Source: CAD feature listing. Evaluate the final solid. Frame: model axes, mm. A direction names the side the tool comes from. Coordinates: 2 decimals unless noted, no trailing zeros. Write each loop counter-clockwise with the first axis right and the second up, starting at its lowest first coordinate (ties: lowest second). Pieces come first, ordered by that corner, then holes. Notation, with made-up numbers: M 44,9.5 L 98,9.5 A15 cw 98,22.5 Z; hole C 22.25,-19 d1. An arc over 180 degrees is marked long. Answer as CSV lines item,"result". Start each with the question number.
1. Section C-C on y = -10. Return the cut outline in (x, z), plus the area to 3 significant figures.
2. Line query: probe 1 along Y at (x, z) = (-26, -24); probe 2 along X at (y, z) = (-25, -14.5); probe 3 along X at (y, z) = (11, -19.5). Output: solid intervals per line, ascending. Write a range as [from, to].
3. Contact query for flat-ended pins moving along their axis: pin 1 Ø1.5 at (x, z) = (12, 3) entering from -Y; pin 2 Ø7 at (x, y) = (-24.5, -17.5) entering from +Z; pin 3 Ø3 at (y, z) = (11.5, -17.5) entering from +X. Output: stop coordinate, or through.
4. Section D-D on z = -43.5. Return the cut outline in (x, y), plus the area to 3 significant figures.
5. Section A-A on z = -24. Return the cut outline in (x, y), plus the area to 3 significant figures.
6. Reachability of faces 5 (the face through (0, 4, -50)), 6 (the face through (-20.5, -26.3, -24.1)), 7 (the face through (50, 3, 6.5)), 8 (the face through (-37.5, 10, -24)) from +Z, -Z, +X, -X, +Y, -Y: full face, straight path, thin tool, end or side. Return the list, or none.
7. Mould query, pull axis Y, two halves, no side actions, for faces 1 (the face through (-31, -26, -28)), 2 (the face through (10, 0, -2)), 3 (the face through (-40.5, 7, -21)), 4 (the face through (1, 5, -13)). Classes: pulls with the +Y half, pulls with the -Y half, needs draft (parallel to the pull), parting line crosses it, or undercut.
8. Section B-B on x = 54. Return the cut outline in (y, z).
```python
from build123d import *

# Parameters (mm, degrees)
EXTRUDE_1_DEPTH     = 5
SKETCH_2_W          = 20
SKETCH_2_H          = 72
EXTRUDE_2_DEPTH     = 33
SKETCH_3_R          = 3
CUT_EXTRUDE_1_DEPTH = 30
SKETCH_4_R          = 5
CUT_EXTRUDE_2_DEPTH = 17
EXTRUDE_START       = 3
SKETCH_5_R          = 5
EXTRUDE_3_DEPTH     = 3
EXTRUDE_4_DEPTH     = 3
EXTRUDE_5_DEPTH     = 10
SKETCH_8_W          = 42
SKETCH_8_H          = 5
EXTRUDE_6_DEPTH     = 25
CUT_EXTRUDE_3_DEPTH = 10
SKETCH_10_W         = 75
SKETCH_10_H         = 0.5
CUT_EXTRUDE_4_DEPTH = 0.5
SKETCH_11_W         = 0.5
SKETCH_11_H         = 15
SKETCH_11_H_2       = 48
CUT_EXTRUDE_5_DEPTH = 0.5


with BuildPart() as part:
    # 草图1 → 凸台-拉伸1 (new body)
    with BuildSketch(Plane(origin=(0, 0, 0), x_dir=(1, 0, 0), z_dir=(0, 1, 0))):
        Polygon((-37.5, 76), (-37.5, -26), (37.5, -26), (37.5, 16), (0, 16), (0, 76), align=None)
    extrude(amount=EXTRUDE_1_DEPTH)

    # 草图2 → 凸台-拉伸2 (add)
    with BuildSketch(Plane.XZ):
        with Locations((-27.5, -40)):
            Rectangle(SKETCH_2_W, SKETCH_2_H)
    extrude(amount=EXTRUDE_2_DEPTH)

    # 草图3 → 切除-拉伸1 (cut)
    with BuildSketch(Plane.ZY.offset(37.5)):
        with Locations((-56, -23)):
            Circle(SKETCH_3_R)
        with Locations((-24, -23)):
            Circle(SKETCH_3_R)
    extrude(amount=-CUT_EXTRUDE_1_DEPTH, mode=Mode.SUBTRACT)

    # 草图4 → 切除-拉伸2 (cut)
    with BuildSketch(Plane.ZY.offset(37.5)):
        with Locations((-56, -23)):
            Circle(SKETCH_4_R)
        with Locations((-24, -23)):
            Circle(SKETCH_4_R)
    extrude(amount=-CUT_EXTRUDE_2_DEPTH, mode=Mode.SUBTRACT)

    # 草图5 → 凸台-拉伸3 (add)
    with BuildSketch(Plane.ZY.offset(37.5).offset(EXTRUDE_START)):
        Polygon((-76, 5), (26, 5), (26, 0), (-4, 0), (-4, -33), (-76, -33), align=None)
        with Locations((-56, -23)):
            Circle(SKETCH_5_R, mode=Mode.SUBTRACT)
        with Locations((-24, -23)):
            Circle(SKETCH_5_R, mode=Mode.SUBTRACT)
    extrude(amount=-EXTRUDE_3_DEPTH)

    # 草图6 → 凸台-拉伸4 (add)
    with BuildSketch(Plane(origin=(0, 0, -76), x_dir=(-1, 0, 0), z_dir=(0, 0, -1))):
        Polygon((0, 5), (0, 0), (17.5, 0), (17.5, -33), (40.5, -33), (40.5, 5), align=None)
    extrude(amount=EXTRUDE_4_DEPTH)

    # 草图7 → 凸台-拉伸5 (add)
    with BuildSketch(Plane(origin=(0, 5, 0), x_dir=(1, 0, 0), z_dir=(0, 1, 0))):
        Polygon((0, 76), (0, 79), (-40.5, 79), (-40.5, -26), (-37.5, -26), (-37.5, 76), align=None)
    extrude(amount=EXTRUDE_5_DEPTH)

    # 草图8 → 凸台-拉伸6 (add)
    with BuildSketch(Plane(origin=(37.5, 0, 0), x_dir=(0, 0, -1), z_dir=(1, 0, 0))):
        with Locations((-5, 2.5)):
            Rectangle(SKETCH_8_W, SKETCH_8_H)
    extrude(amount=EXTRUDE_6_DEPTH)

    # 草图9 → 切除-拉伸3 (cut)
    with BuildSketch(Plane(origin=(0, 5, 0), x_dir=(1, 0, 0), z_dir=(0, 1, 0))):
        with BuildLine():
            Line((57.5, -3.5), (42.5, -3.5))
            ThreePointArc((42.5, -3.5), (41, -5), (42.5, -6.5))
            Line((42.5, -6.5), (57.5, -6.5))
            ThreePointArc((57.5, -6.5), (59, -5), (57.5, -3.5))
        make_face()
    extrude(amount=-CUT_EXTRUDE_3_DEPTH, mode=Mode.SUBTRACT)

    # 草图10 → 切除-拉伸4 (cut)
    with BuildSketch(Plane.ZY.offset(40.5)):
        with Locations((-41.5, -0.25)):
            Rectangle(SKETCH_10_W, SKETCH_10_H)
    extrude(amount=-CUT_EXTRUDE_4_DEPTH, mode=Mode.SUBTRACT)

    # 草图11 → 切除-拉伸5 (cut)
    with BuildSketch(Plane.ZY.offset(40.5)):
        with Locations((-3.75, 7.5)):
            Rectangle(SKETCH_11_W, SKETCH_11_H)
        with Locations((-38.75, -9)):
            Rectangle(SKETCH_11_W, SKETCH_11_H_2)
    extrude(amount=-CUT_EXTRUDE_5_DEPTH, mode=Mode.SUBTRACT)


solid = part.part
```
Values:
1,outline,"M -40.5,-79 L -17.5,-79 L -17.5,-4 L -40.5,-4 L -40.5,-38.5 L -40,-38.5 L -40,-39 L -40.5,-39 Z"
1,area,"1,720 mm²"
2,probe 1,"[-33, -28], [-18, 5]"
2,probe 2,"[-40.5, -17.5]"
2,probe 3,"[-40.5, -37.5]"
3,pin 1,"y = 0"
3,pin 2,"z = -4"
3,pin 3,"x = -37.5"
4,outline,"M -40.5,-33 L -17.5,-33 L -17.5,0 L 0,0 L 0,5 L -37.5,5 L -37.5,15 L -40.5,15 L -40.5,0 L -40,0 L -40,-0.5 L -40.5,-0.5 Z"
4,area,"991 mm²"
5,outline,"M -40.5,-33 L -17.5,-33 L -17.5,-26 L -20.5,-26 L -20.5,-28 L -40.5,-28 Z; M -40.5,-18 L -20.5,-18 L -20.5,-20 L -17.5,-20 L -17.5,0 L 0,0 L 0,5 L -37.5,5 L -37.5,15 L -40.5,15 L -40.5,0 L -40,0 L -40,-0.5 L -40.5,-0.5 Z"
5,area,"773 mm²"
6,face 5,"-Z, +X, +Y, -Y"
6,face 6,"-X"
6,face 7,"+Y, -Y"
6,face 8,"+Z, +X, +Y"
7,face 1,"undercut"
7,face 2,"pulls with the -Y half"
7,face 3,"needs draft"
7,face 4,"pulls with the +Y half"
8,outline,"M 0,-16 L 5,-16 L 5,3.5 L 0,3.5 Z; M 0,6.5 L 5,6.5 L 5,26 L 0,26 Z"
